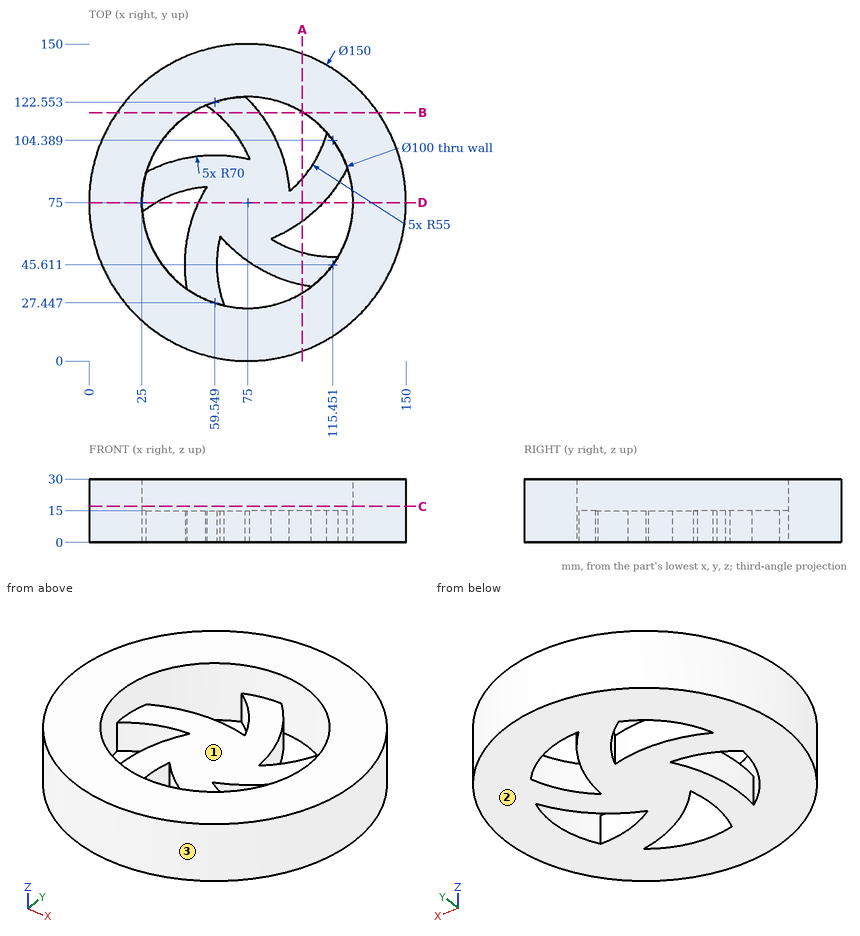
Check sheet for the drawn part. Datum: minimum x, y, z corner. Units: mm. Round coordinates to 2 decimals unless told otherwise and drop trailing zeros. Order: outer loops, then holes, each group sorted by start corner. A loop starts at its lowest first (then second) coordinate and runs counter-clockwise, first axis right, second up. Notation, with made-up numbers: M 19,49.25 L 34,49.25 A12 ccw 34,60.25 Z; hole C -37,19 d9. An arc over 180 degrees is marked long. Answer in a Markdown table with one row per item.
(1) Gauge pin test, flat ends, axial feed: pin 1 (2 mm diameter, centred on x = 95.5, z = 10.5, fed in from -Y); pin 2 (4 mm diameter, centred on y = 35.5, z = 17, fed in from +X); pin 3 (1.5 mm diameter, centred on y = 127, z = 25, fed in from -X); pin 4 (2 mm diameter, centred on x = 70, y = 27.5, fed in from +Z) (3 decimals). Record the tip position at first contact, or that the pin passes through.
Findings:
| item | result |
|---|---|
| pin 1 | stops at y = 2.58 |
| pin 2 | stops at x = 139.95 |
| pin 3 | stops at x = 20.24 |
| pin 4 | passes through |
(2) Draft check along Z on the marked faces 1, 2 and 3. Enter one of: +Z half, -Z half, draft (parallel to the pull), parting line (faces both ways), or undercut.
Findings:
| item | result |
|---|---|
| face 1 | +Z half |
| face 2 | -Z half |
| face 3 | draft |
(3) Section check A-A on x = 101. Record the boundary of the cut face in (y, z) (1 decimal).
Findings:
| item | result |
|---|---|
| outline | M 4.7,0 L 32.3,0 L 32.3,30 L 4.7,30 Z; M 35.9,0 L 51.3,0 L 51.3,15 L 35.9,15 Z; M 66.1,0 L 86.4,0 L 86.4,15 L 66.1,15 Z; M 117.7,0 L 145.3,0 L 145.3,30 L 117.7,30 Z |
(4) Section check D-D on y = 75. Record the boundary of the cut face in (x, z), plus the area to 3 significant figures.
Findings:
| item | result |
|---|---|
| outline | M 0,0 L 31.91,0 L 31.91,15 L 25,15 L 25,30 L 0,30 Z; M 51.92,0 L 110.92,0 L 110.92,15 L 51.92,15 Z; M 125,0 L 150,0 L 150,30 L 125,30 Z |
| area | 2,490 mm^2 |
(5) Material ranges on line 1 along Y through (x, z) = (75, 22); line 2 along Y through (x, z) = (75, 7.25) (1 decimal); line 3 along X through (y, z) = (117.5, 9.25) (1 decimal), recorded low to high. Write a range as from..to.
Findings:
| item | result |
|---|---|
| line 1 | y = 0..25, 125..150 |
| line 2 | y = 0..25, 47.3..95.7, 97.9..124, 125..150 |
| line 3 | x = 13.2..48.7, 59.9..80.6, 101.3..136.8 |
(6) Section check C-C on z = 17. Record the boundary of the cut face in (x, y), plus the area to 3 significant figures.
Findings:
| item | result |
|---|---|
| outline | C 75,75 d150; hole C 75,75 d100 |
| area | 9,820 mm^2 |
(7) Section check B-B on y = 117.5. Record the boundary of the cut face in (x, z), plus the area to 3 significant figures.
Findings:
| item | result |
|---|---|
| outline | M 13.2,0 L 48.66,0 L 48.66,30 L 13.2,30 Z; M 59.91,0 L 80.62,0 L 80.62,15 L 59.91,15 Z; M 101.34,0 L 136.8,0 L 136.8,30 L 101.34,30 Z |
| area | 2,440 mm^2 |
